Work out the finished part from the listing and answer in its coordinate system (mm). A direction names the side the tool comes from. Round coordinates to 2 decimals unless told otherwise and drop trailing zeros. Order: outer loops, then holes, each group sorted by start corner. A loop starts at its lowest first (then second) coordinate and runs counter-clockwise, first axis right, second up. Notation, with made-up numbers: (-5, 43) - (40, 43) arc R9 cw to (40, 57) - close; hole circle Ø11 at (56.5, 55). An arc over 180 degrees is marked (long way). Answer in a Markdown table with one row per item.
from build123d import *

# Parameters (mm, degrees)
F0_R     = 10.9728
F1_DEPTH = 21.7805
F2_R     = 0.7747
F3_DEPTH = 6.35
F5_DEPTH = 1.8669
F6_R     = 2.01295
F7_DEPTH = 2.54
F8_W     = 15.367
F8_H     = 13.295026
F9_DEPTH = 31.9786


with BuildPart() as f1:
    # F0 (on Top) → F1 (new body)
    with BuildSketch(Plane.XY):
        with Locations((-29.485371, 20.489834)):
            Circle(F0_R)
    extrude(amount=F1_DEPTH)

    # F2 (on face) → F3 (cut)
    with BuildSketch(Plane.XY.offset(21.7805)):
        with Locations((-38.438871, 20.489834)):
            Circle(F2_R)
        with Locations((-29.485371, 11.536334)):
            Circle(F2_R)
        with Locations((-20.531871, 20.489834)):
            Circle(F2_R)
        with Locations((-29.485371, 29.443334)):
            Circle(F2_R)
    extrude(amount=-F3_DEPTH, mode=Mode.SUBTRACT)

    # F4 (on face) → F5 (join)
    with BuildSketch(Plane.XY.offset(21.7805)):
        with BuildLine():
            Line((-32.999739, 14.482734), (-25.971003, 14.482734))
            ThreePointArc((-25.971003, 14.482734), (-22.525771, 20.489834), (-25.971003, 26.496934))
            Line((-25.971003, 26.496934), (-32.999739, 26.496934))
            ThreePointArc((-32.999739, 26.496934), (-36.444971, 20.489834), (-32.999739, 14.482734))
        make_face()
    extrude(amount=F5_DEPTH)

    # F6 (on face) → F7 (cut)
    with BuildSketch(Plane.XY.offset(23.6474)):
        with Locations((-29.485371, 20.489834)):
            Circle(F6_R)
    extrude(amount=-F7_DEPTH, mode=Mode.SUBTRACT)

    # F8 (on face) → F9 (join)
    with BuildSketch(Plane(origin=(0, 0, 0), x_dir=(1, 0, 0), z_dir=(0, 0, -1))):
        with BuildLine():
            ThreePointArc((-37.168871, -27.137347), (-29.485371, -30.649834), (-21.801871, -27.137347))
            Line((-21.801871, -27.137347), (-37.168871, -27.137347))
        make_face()
        with Locations((-29.485371, -20.489834)):
            Rectangle(F8_W, F8_H)
        with BuildLine():
            Line((-37.168871, -13.842321), (-21.801871, -13.842321))
            ThreePointArc((-21.801871, -13.842321), (-29.485371, -10.329834), (-37.168871, -13.842321))
        make_face()
    extrude(amount=F9_DEPTH)


solid = f1.part
1) Find section A-A, the plane y = 17.5. Give the vertices of the cut face in (x, z).
Filled in:
| item | result |
|---|---|
| outline | (-40.04, 0) - (-37.17, 0) - (-37.17, -31.98) - (-21.8, -31.98) - (-21.8, 0) - (-18.93, 0) - (-18.93, 21.78) - (-23.2, 21.78) - (-23.2, 23.65) - (-35.77, 23.65) - (-35.77, 21.78) - (-40.04, 21.78) - close |
2) The mould has two halves that part along X. Classify faces 1 (the face through (-30.91, 31.37, 10.74)), 2 (the face through (-21.802, 21, -16)), 3 (the face through (-30, 14.483, 23)), 4 (the face through (-30, 21, 21.107)): released by +X, released by -X, zero draft, split by the parting line, or undercut.
Filled in:
| item | result |
|---|---|
| face 1 | split by the parting line |
| face 2 | released by +X |
| face 3 | zero draft |
| face 4 | undercut |
3) Find section C-C, the plane z = 13. Give the vertices of the cut face in (x, y).
Filled in:
| item | result |
|---|---|
| outline | circle Ø21.95 at (-29.49, 20.49) |
4) Find the intervals of material crossed by probe 1 along Y at (x, z) = (-35.5, -25.5); probe 2 along Z at (x, y) = (-30, 19.5); probe 3 along X at (y, z) = (23, -6), in increasing order. Write a range as from..to.
Filled in:
| item | result |
|---|---|
| probe 1 | y = 12.3..28.68 |
| probe 2 | z = -31.98..21.11 |
| probe 3 | x = -37.17..-21.8 |
5) Which of the six approach directions +Z, -Z, +X, -X, +Y, -Y give full straight-line access (tool end or side, diameter ignored) to faces 5 (the face through (-35, 26, 21.78)), 6 (the face through (-29.61, 30.65, -15.77)), 7 (the face through (-36.444, 20.591, 22.701)), 8 (the face through (-37.169, 21, -16)), 9 (the face through (-21, 21, 0))?
Filled in:
| item | result |
|---|---|
| face 5 | +Z |
| face 6 | -Z, +Y |
| face 7 | +Z, -X |
| face 8 | -Z, -X, +Y, -Y |
| face 9 | -Z |
6) Each of these flat-tipped pins is pushed along its axis until it touches: pin 1 (0.8 mm diameter, centred on x = -29.5, y = 11.5, fed in from +Z); pin 2 (8 mm diameter, centred on x = -37, z = -2, fed in from -Y); pin 3 (4 mm diameter, centred on y = 20, z = -21.5, fed in from -X); pin 4 (10 mm diameter, centred on y = 22, z = 16.5, fed in from +X). Where does it stop, or does it pass through?
Filled in:
| item | result |
|---|---|
| pin 1 | stops at z = 15.43 |
| pin 2 | stops at y = 10.29 |
| pin 3 | stops at x = -37.17 |
| pin 4 | stops at x = -18.51 |
7) Find section B-B, the plane z = -25. Give the vertices of the cut face in (x, y).
Filled in:
| item | result |
|---|---|
| outline | (-37.17, 13.84) arc R10.16 ccw to (-21.8, 13.84) - (-21.8, 27.14) arc R10.16 ccw to (-37.17, 27.14) - close |
